```python
from build123d import *

# Parameters (mm, degrees)
PAD008_DEPTH    = 9.5
SKETCH017_W     = 3
SKETCH017_H     = 10
POCKET002_DEPTH = 7.5
POCKET003_DEPTH = 0.7
POCKET004_DEPTH = 0.7
CHAMFER001_SIZE = 0.6
FILLET002_R     = 0.65
SKETCH014_R     = 1.05
POCKET005_DEPTH = 2
POCKET006_DEPTH = 8
SKETCH022_R     = 2.5375
POCKET007_DEPTH = 8.736873
SKETCH021_R     = 5.575
POCKET008_DEPTH = 1.236873
SKETCH024_R     = 6.075
POCKET009_DEPTH = 6.1
SKETCH025_R     = 5
POCKET010_DEPTH = 8.736873
SKETCH015_R     = 0.75
POCKET011_DEPTH = 8.736873


with BuildPart() as part:
    # Sketch016 → Pad008 (new body, symmetric)
    with BuildSketch(Plane.YZ):
        with BuildLine():
            ThreePointArc((20.3007, 8.33036), (0, 8.735873), (-20.3007, 8.33036))
            Line((-20.3007, 8.33036), (-20.59728, 0))
            Line((20.59728, 0), (-20.59728, 0))
            Line((20.3007, 8.33036), (20.59728, 0))
        make_face()
    extrude(amount=PAD008_DEPTH, both=True)

    # Sketch017 → Pocket002 (cut, symmetric)
    with BuildSketch(Plane.YZ):
        with Locations((21.175, 5)):
            Rectangle(SKETCH017_W, SKETCH017_H)
        with Locations((-21.175, 5)):
            Rectangle(SKETCH017_W, SKETCH017_H)
    extrude(amount=POCKET002_DEPTH, both=True, mode=Mode.SUBTRACT)

    # Sketch018 → Pocket003 (cut, symmetric)
    with BuildSketch(Plane.YZ.offset(6.8)):
        Polygon((-19.925, 8.9), (-11.553945, 8.9), (-18.398945, -9.9), (-19.925, -9.9), align=None)
        Polygon((19.925, 8.9), (11.553945, 8.9), (18.398945, -9.9), (19.925, -9.9), align=None)
    extrude(amount=POCKET003_DEPTH, both=True, mode=Mode.SUBTRACT)

    # Sketch019 → Pocket004 (cut, symmetric)
    with BuildSketch(Plane.YZ.offset(-6.8)):
        Polygon((-19.925, 8.9), (-11.553945, 8.9), (-18.398945, -9.9), (-19.925, -9.9), align=None)
        Polygon((19.925, 8.9), (11.553945, 8.9), (18.398945, -9.9), (19.925, -9.9), align=None)
    extrude(amount=POCKET004_DEPTH, both=True, mode=Mode.SUBTRACT)

    # Chamfer001
    chamfer001_edges = [part.edges().sort_by_distance(p)[0] for p in [
        (9.5, 20.44899, 4.16518),
        (9.5, -20.44899, 4.16518),
        (-9.5, -20.44899, 4.16518),
        (-9.5, 20.44899, 4.16518),
    ]]
    chamfer(chamfer001_edges, length=CHAMFER001_SIZE)

    # Fillet002
    fillet002_edges = [part.edges().sort_by_distance(p)[0] for p in [
        (7.5, 13.228407, 4.301038),
        (7.5, -13.228407, 4.301038),
        (-6.1, -13.228407, 4.301038),
        (-6.1, 13.228407, 4.301038),
        (-7.5, -13.228407, 4.301038),
        (6.1, -13.228407, 4.301038),
        (6.1, 13.228407, 4.301038),
        (-7.5, 13.228407, 4.301038),
    ]]
    fillet(fillet002_edges, radius=FILLET002_R)

    # Sketch014 → Pocket005 (cut)
    with BuildSketch(Plane.XY):
        with Locations((7.25, 10.4875)):
            Circle(SKETCH014_R)
        with Locations((7.25, 12.9875)):
            Circle(SKETCH014_R)
        with BuildLine():
            ThreePointArc((5.7075, 6.5725), (4.5575, 5.4225), (5.7075, 4.2725))
            Line((5.7075, 4.2725), (7.5075, 4.2725))
            ThreePointArc((7.5075, 4.2725), (8.6575, 5.4225), (7.5075, 6.5725))
            Line((7.5075, 6.5725), (5.7075, 6.5725))
        make_face()
        with BuildLine():
            ThreePointArc((7.8, -5.15), (6.95, -6), (7.8, -6.85))
            Line((7.8, -6.85), (8.35, -6.85))
            ThreePointArc((8.35, -6.85), (9.2, -6), (8.35, -5.15))
            Line((8.35, -5.15), (7.8, -5.15))
        make_face()
        with BuildLine():
            ThreePointArc((5.0575, 2.7625), (4.703947, 2.616053), (4.5575, 2.2625))
            Line((4.5575, 0.9625), (4.5575, 2.2625))
            ThreePointArc((4.5575, 0.9625), (4.703947, 0.608947), (5.0575, 0.4625))
            Line((8.1575, 0.4625), (5.0575, 0.4625))
            ThreePointArc((8.1575, 0.4625), (8.511053, 0.608947), (8.6575, 0.9625))
            Line((8.6575, 2.2625), (8.6575, 0.9625))
            ThreePointArc((8.6575, 2.2625), (8.511053, 2.616053), (8.1575, 2.7625))
            Line((5.0575, 2.7625), (8.1575, 2.7625))
        make_face()
        with BuildLine():
            ThreePointArc((7.45, -3.15), (7.096447, -3.296447), (6.95, -3.65))
            Line((6.95, -4.35), (6.95, -3.65))
            ThreePointArc((6.95, -4.35), (7.096447, -4.703553), (7.45, -4.85))
            Line((8.7, -4.85), (7.45, -4.85))
            ThreePointArc((8.7, -4.85), (9.053553, -4.703553), (9.2, -4.35))
            Line((9.2, -3.65), (9.2, -4.35))
            ThreePointArc((9.2, -3.65), (9.053553, -3.296447), (8.7, -3.15))
            Line((7.45, -3.15), (8.7, -3.15))
        make_face()
    extrude(amount=POCKET005_DEPTH, mode=Mode.SUBTRACT)

    # Sketch020 → Pocket006 (cut)
    with BuildSketch(Plane.XY):
        with BuildLine():
            ThreePointArc((2.625, 1.290349), (-2.925, 0), (2.625, -1.290349))
            Line((2.625, -1.290349), (2.625, 1.290349))
        make_face()
    extrude(amount=POCKET006_DEPTH, mode=Mode.SUBTRACT)

    # Sketch022 → Pocket007 (cut, through all)
    with BuildSketch(Plane.XY):
        Circle(SKETCH022_R)
    extrude(amount=POCKET007_DEPTH, mode=Mode.SUBTRACT)

    # Sketch021 → Pocket008 (cut, through all)
    with BuildSketch(Plane.XY.offset(7.5)):
        with Locations((0, -11)):
            Circle(SKETCH021_R)
    extrude(amount=POCKET008_DEPTH, mode=Mode.SUBTRACT)

    # Cone → Cone (revolve, cut)
    with BuildSketch(Plane(origin=(0, -11, 0), x_dir=(0, 1, 0), z_dir=(1, 0, 0))):
        Polygon((0, 0), (3.5, 0), (5, 10), (0, 10), align=None)
    revolve(axis=Axis((0, -11, 0), (0, 0, 1)), mode=Mode.SUBTRACT)

    # Sketch024 → Pocket009 (cut)
    with BuildSketch(Plane.XY):
        with Locations((0, 11)):
            Circle(SKETCH024_R)
    extrude(amount=POCKET009_DEPTH, mode=Mode.SUBTRACT)

    # Sketch025 → Pocket010 (cut, through all)
    with BuildSketch(Plane.XY):
        with Locations((0, 11)):
            Circle(SKETCH025_R)
    extrude(amount=POCKET010_DEPTH, mode=Mode.SUBTRACT)

    # Sketch015 → Pocket011 (cut, through all)
    with BuildSketch(Plane.XY):
        with Locations((-8.125, 12)):
            Circle(SKETCH015_R)
        with Locations((8.125, -12)):
            Circle(SKETCH015_R)
    extrude(amount=POCKET011_DEPTH, mode=Mode.SUBTRACT)


with BuildPart() as part_1:
    # Body005 placement: moved
    add(part.part.moved(Location((0, 0, 1.9))))


solid = part_1.part
```
Verification items for the finished model (mm, model axes). A direction names the side the tool comes from. Give positions to 0.01 mm unless a question says otherwise; leave off trailing zeros. Order: outer loops, then holes, each group sorted by start corner. A loop starts at its lowest first (then second) coordinate and runs counter-clockwise, first axis right, second up. Notation, with made-up numbers: M -29.75,84 L 8.25,84 A18 cw 8.25,115 Z; hole C 84,71 d4. An arc over 180 degrees is marked long. Answer in a Markdown table with one row per item. Add a question column.
Item 1: Section check B-B, the plane y = 18. Enter the section's corners in (x, z), and give its area (3 significant figures).
Item 2: Gauge pin test, flat ends, axial feed: pin 1 (0.7 mm diameter, centred on x = 7, y = 2, fed in from -Z); pin 2 (2 mm diameter, centred on x = 3.5, z = 7, fed in from +Y) (3 decimals); pin 3 (0.5 mm diameter, centred on x = 7, z = 3, fed in from -Y). Record the tip position at first contact, or that the pin passes through.
Item 3: Mould release check, pull along Y, two halves, no side actions. Record for faces 6 (the flat face through (-5, 13, 8)), 7 (the cylindrical face through (-1.08, 6.12, 9.28)), 8 (the flat face through (7.5, -17, 6)), 9 (the cylindrical face through (7.305, 13.466, 6.091)): released by +Y, released by -Y, zero draft, split by the parting line, or undercut.
Item 4: Scan lines: probe 1 along Y at (x, z) = (0, 10.15) (1 decimal); probe 2 along X at (y, z) = (11, 10.15); probe 3 along X at (y, z) = (-11.5, 7.5). Record each from-to range of solid material in increasing order. Write a range as from..to.
Item 5: Section check D-D, the plane y = -6. Enter the section's corners in (x, z).
Item 6: Section check A-A, the plane x = 0. State how many separate pieces and enclosed holes the cut face has, and give its area (3 significant figures).
Item 7: Tool access check on faces 1 (the flat face through (0, 19.675, 6)), 2 (the cylindrical face through (6.285, 13.475, 6.095)), 3 (the flat face through (-9.5, 0, 6)), 4 (the cylindrical face through (4.558, 5.448, 2.886)), 5 (the flat face through (1, -6, 9.4)). Record the directions out of +Z, -Z, +X, -X, +Y, -Y that give a thin tool (end or side, any length) a straight path to the whole face; none if there is none.
Filled sheet:
| question | item | result |
|---|---|---|
| 1 | outline | M -9.5,1.9 L -7.5,1.9 L -7.5,10.32 L -9.5,10.32 Z; M -6.1,1.9 L 6.1,1.9 L 6.1,10.32 L -6.1,10.32 Z; M 7.5,1.9 L 9.5,1.9 L 9.5,10.32 L 7.5,10.32 Z |
| 1 | area | 136 mm^2 |
| 2 | pin 1 | stops at z = 3.9 |
| 2 | pin 2 | stops at y = 19.675 |
| 2 | pin 3 | stops at y = -14.56 |
| 3 | face 6 | undercut |
| 3 | face 7 | undercut |
| 3 | face 8 | zero draft |
| 3 | face 9 | released by +Y |
| 4 | probe 1 | y = -19.7..-16.6, -5.4..-2.5, 2.5..6, 16..19.7 |
| 4 | probe 2 | x = -9.5..-5, 5..9.5 |
| 4 | probe 3 | x = -9.5..-4.31, 4.31..7.57, 8.68..9.5 |
| 5 | outline | M -9.5,1.9 L 6.95,1.9 L 6.95,3.9 L 9.2,3.9 L 9.2,1.9 L 9.5,1.9 L 9.5,10.6 L 2.47,10.6 L 2.47,9.4 L -2.47,9.4 L -2.47,10.6 L -9.5,10.6 Z |
| 6 | separate pieces | 4 |
| 6 | enclosed holes | 0 |
| 6 | area | 116 mm^2 |
| 7 | face 1 | +Z, -Z, +Y |
| 7 | face 2 | +Z, +Y |
| 7 | face 3 | +Z, -Z, -X, +Y, -Y |
| 7 | face 4 | -Z |
| 7 | face 5 | +Z |
